Work out the finished part from the listing and answer in its coordinate system (mm). A direction names the side the tool comes from. Give positions to 0.01 mm unless a question says otherwise; leave off trailing zeros. Loops run counter-clockwise (first coordinate to the right, second up) from the corner with the lowest first, then second, coordinate; pieces in that order, holes last. Notation, with made-up numbers: M 3.5,-17.75 L 34.5,-17.75 A32 cw 34.5,11.25 Z; hole C 36.5,52.5 d1. An arc over 180 degrees is marked long. Answer in a Markdown table with one row per item. Add a question column.
from build123d import *

# Parameters (mm, degrees)
SKETCH_1_W          = 250
SKETCH_1_H          = 250
EXTRUDE_1_DEPTH     = 5.8
CUT_EXTRUDE_1_REACH = 355.601
SKETCH_2_W          = 53
SKETCH_2_H          = 5.8
SKETCH_2_W_2        = 5.8
SKETCH_2_H_2        = 47.2


with BuildPart() as part:
    # Эскиз1 → Бобышка-Вытянуть1 (new body)
    with BuildSketch(Plane(origin=(0, 0, 0), x_dir=(1, 0, 0), z_dir=(0, 1, 0))):
        with Locations((125, 125)):
            Rectangle(SKETCH_1_W, SKETCH_1_H)
    extrude(amount=EXTRUDE_1_DEPTH)

    # Эскиз2 → Вырез-Вытянуть1 (cut, up to next)
    with BuildSketch(Plane.XZ, mode=Mode.PRIVATE) as cut_extrude_1_sk1:
        with Locations((74.5, -2.9)):
            Rectangle(SKETCH_2_W, SKETCH_2_H)
    cut_extrude_1_tool1 = extrude(cut_extrude_1_sk1.sketch, amount=-CUT_EXTRUDE_1_REACH, mode=Mode.PRIVATE) & part.part
    # Эскиз2 → Вырез-Вытянуть1 (cut, up to next)
    with BuildSketch(Plane.XZ, mode=Mode.PRIVATE) as cut_extrude_1_sk2:
        with Locations((175.5, -2.9)):
            Rectangle(SKETCH_2_W, SKETCH_2_H)
    cut_extrude_1_tool2 = extrude(cut_extrude_1_sk2.sketch, amount=-CUT_EXTRUDE_1_REACH, mode=Mode.PRIVATE) & part.part
    # Эскиз2 → Вырез-Вытянуть1 (cut, up to next)
    with BuildSketch(Plane.XZ, mode=Mode.PRIVATE) as cut_extrude_1_sk3:
        with Locations((125, -77.4)):
            Rectangle(SKETCH_2_W_2, SKETCH_2_H_2)
    cut_extrude_1_tool3 = extrude(cut_extrude_1_sk3.sketch, amount=-CUT_EXTRUDE_1_REACH, mode=Mode.PRIVATE) & part.part
    # Эскиз2 → Вырез-Вытянуть1 (cut, up to next)
    with BuildSketch(Plane.XZ, mode=Mode.PRIVATE) as cut_extrude_1_sk4:
        with Locations((2.9, -77.4)):
            Rectangle(SKETCH_2_W_2, SKETCH_2_H_2)
    cut_extrude_1_tool4 = extrude(cut_extrude_1_sk4.sketch, amount=-CUT_EXTRUDE_1_REACH, mode=Mode.PRIVATE) & part.part
    # Эскиз2 → Вырез-Вытянуть1 (cut, up to next)
    with BuildSketch(Plane.XZ, mode=Mode.PRIVATE) as cut_extrude_1_sk5:
        with Locations((2.9, -172.6)):
            Rectangle(SKETCH_2_W_2, SKETCH_2_H_2)
    cut_extrude_1_tool5 = extrude(cut_extrude_1_sk5.sketch, amount=-CUT_EXTRUDE_1_REACH, mode=Mode.PRIVATE) & part.part
    # Эскиз2 → Вырез-Вытянуть1 (cut, up to next)
    with BuildSketch(Plane.XZ, mode=Mode.PRIVATE) as cut_extrude_1_sk6:
        with Locations((125, -172.6)):
            Rectangle(SKETCH_2_W_2, SKETCH_2_H_2)
    cut_extrude_1_tool6 = extrude(cut_extrude_1_sk6.sketch, amount=-CUT_EXTRUDE_1_REACH, mode=Mode.PRIVATE) & part.part
    # Эскиз2 → Вырез-Вытянуть1 (cut, up to next)
    with BuildSketch(Plane.XZ, mode=Mode.PRIVATE) as cut_extrude_1_sk7:
        with Locations((74.5, -247.1)):
            Rectangle(SKETCH_2_W, SKETCH_2_H)
    cut_extrude_1_tool7 = extrude(cut_extrude_1_sk7.sketch, amount=-CUT_EXTRUDE_1_REACH, mode=Mode.PRIVATE) & part.part
    # Эскиз2 → Вырез-Вытянуть1 (cut, up to next)
    with BuildSketch(Plane.XZ, mode=Mode.PRIVATE) as cut_extrude_1_sk8:
        with Locations((175.5, -247.1)):
            Rectangle(SKETCH_2_W, SKETCH_2_H)
    cut_extrude_1_tool8 = extrude(cut_extrude_1_sk8.sketch, amount=-CUT_EXTRUDE_1_REACH, mode=Mode.PRIVATE) & part.part
    # Эскиз2 → Вырез-Вытянуть1 (cut, up to next)
    with BuildSketch(Plane.XZ, mode=Mode.PRIVATE) as cut_extrude_1_sk9:
        with Locations((247.1, -172.6)):
            Rectangle(SKETCH_2_W_2, SKETCH_2_H_2)
    cut_extrude_1_tool9 = extrude(cut_extrude_1_sk9.sketch, amount=-CUT_EXTRUDE_1_REACH, mode=Mode.PRIVATE) & part.part
    # Эскиз2 → Вырез-Вытянуть1 (cut, up to next)
    with BuildSketch(Plane.XZ, mode=Mode.PRIVATE) as cut_extrude_1_sk10:
        with Locations((247.1, -77.4)):
            Rectangle(SKETCH_2_W_2, SKETCH_2_H_2)
    cut_extrude_1_tool10 = extrude(cut_extrude_1_sk10.sketch, amount=-CUT_EXTRUDE_1_REACH, mode=Mode.PRIVATE) & part.part
    add(cut_extrude_1_tool1.solids().sort_by_distance((74.5, 0, -2.9))[0], mode=Mode.SUBTRACT)
    add(cut_extrude_1_tool2.solids().sort_by_distance((175.5, 0, -2.9))[0], mode=Mode.SUBTRACT)
    add(cut_extrude_1_tool3.solids().sort_by_distance((125, 0, -77.4))[0], mode=Mode.SUBTRACT)
    add(cut_extrude_1_tool4.solids().sort_by_distance((2.9, 0, -77.4))[0], mode=Mode.SUBTRACT)
    add(cut_extrude_1_tool5.solids().sort_by_distance((2.9, 0, -172.6))[0], mode=Mode.SUBTRACT)
    add(cut_extrude_1_tool6.solids().sort_by_distance((125, 0, -172.6))[0], mode=Mode.SUBTRACT)
    add(cut_extrude_1_tool7.solids().sort_by_distance((74.5, 0, -247.1))[0], mode=Mode.SUBTRACT)
    add(cut_extrude_1_tool8.solids().sort_by_distance((175.5, 0, -247.1))[0], mode=Mode.SUBTRACT)
    add(cut_extrude_1_tool9.solids().sort_by_distance((247.1, 0, -172.6))[0], mode=Mode.SUBTRACT)
    add(cut_extrude_1_tool10.solids().sort_by_distance((247.1, 0, -77.4))[0], mode=Mode.SUBTRACT)


solid = part.part
(1) Consider line 1 along X through (y, z) = (4.35, -152); line 2 along Z through (x, y) = (187, 0.65). Determine where each line is inside the solid, lowest interval first. Write a range as from..to.
(2) Section A-A, the plane z = -63 is taken. Determine the outline of the cut face in (x, y).
(3) Section B-B, the plane y = 3.9 is taken. State how many separate pieces and enclosed holes the cut face has, and give its area (3 significant figures).
(4) Section C-C, the plane x = 157 is taken. Determine the outline of the cut face in (y, z), and give its area (3 significant figures).
(5) Each of these flat-tipped pins is pushed along its axis until it touches: P1, Ø1.7, axis at y = 2, z = -177.5, coming from the -X side; P2, Ø1.7, axis at x = 63, y = 3, coming from the -Z side; P3, Ø1.7, axis at y = 4, z = -164, coming from the +X side; P4, Ø2, axis at x = 154.5, z = -29.5, coming from the -Y side. Where does it stop, or does it pass through?
(6) The mould has two halves that part along X. Classify faces 6 (the face through (122.1, 3, -78)), 7 (the face through (250, 3, -27)), 8 (the face through (123, 5.8, -127)): pulls with the +X half, pulls with the -X half, needs draft (parallel to the pull), parting line crosses it, or undercut.
(7) Which of the six approach directions +Z, -Z, +X, -X, +Y, -Y give full straight-line access (tool end or side, diameter ignored) to faces 1 (the face through (226, 3, 0)), 2 (the face through (175, 3, -5.8)), 3 (the face through (5.8, 3, -173)), 4 (the face through (127.9, 3, -78)), 5 (the face through (247, 3, -101))?
Numbers:
| question | item | result |
|---|---|---|
| 1 | line 1 | x = 5.8..122.1, 127.9..244.2 |
| 1 | line 2 | z = -244.2..-5.8 |
| 2 | outline | M 5.8,0 L 122.1,0 L 122.1,5.8 L 5.8,5.8 Z; M 127.9,0 L 244.2,0 L 244.2,5.8 L 127.9,5.8 Z |
| 3 | separate pieces | 1 |
| 3 | enclosed holes | 2 |
| 3 | area | 59,600 mm² |
| 4 | outline | M 0,-244.2 L 5.8,-244.2 L 5.8,-5.8 L 0,-5.8 Z |
| 4 | area | 1,380 mm² |
| 5 | P1 | stops at x = 5.8 |
| 5 | P2 | stops at z = -244.2 |
| 5 | P3 | stops at x = 244.2 |
| 5 | P4 | stops at y = 0 |
| 6 | face 6 | undercut |
| 6 | face 7 | pulls with the +X half |
| 6 | face 8 | needs draft |
| 7 | face 1 | +Z, +X, -X, +Y, -Y |
| 7 | face 2 | +Z, +Y, -Y |
| 7 | face 3 | -X, +Y, -Y |
| 7 | face 4 | +Y, -Y |
| 7 | face 5 | +X, +Y, -Y |
